Here's the drawing with two shaded views (mm, measured from the low corner). I have some questions. Round coordinates to 2 decimals unless told otherwise and drop trailing zeros. Loops run counter-clockwise (first coordinate to the right, second up) from the corner with the lowest first, then second, coordinate; pieces in that order, holes last.
(1) If I drill on line 1 along Y through (x, z) = (1.1, 88); line 2 along Y through (x, z) = (3.95, 91); line 3 along Z through (x, y) = (3.9, 36), over which ranges is the centre line in solid material (lowest first)?
(2) I want a section at A-A on z = 31. Write out the boundary of the cut face in (x, y).
(3) I want a section at D-D on y = 28.5. Write out the boundary of the cut face in (x, z).
(4) I want a section at B-B on z = 88. Write out the boundary of the cut face in (x, y), plus the area to 3 significant figures.
(5) Will these pins go through, and if not, where does the flat tip stop? pin 1 Ø1.5 at (x, z) = (2.5, 120.5) entering from -Y; pin 2 Ø5 at (y, z) = (64.5, 38) entering from -X; pin 3 Ø1.5 at (x, y) = (1.5, 77) entering from -Z; pin 4 Ø1.5 at (x, y) = (3.5, 78) entering from +Z.
(6) I want a section at C-C on x = 3.3. Give the number of separate pieces and of enclosed holes in the cut face, plus the area to 3 significant figures.
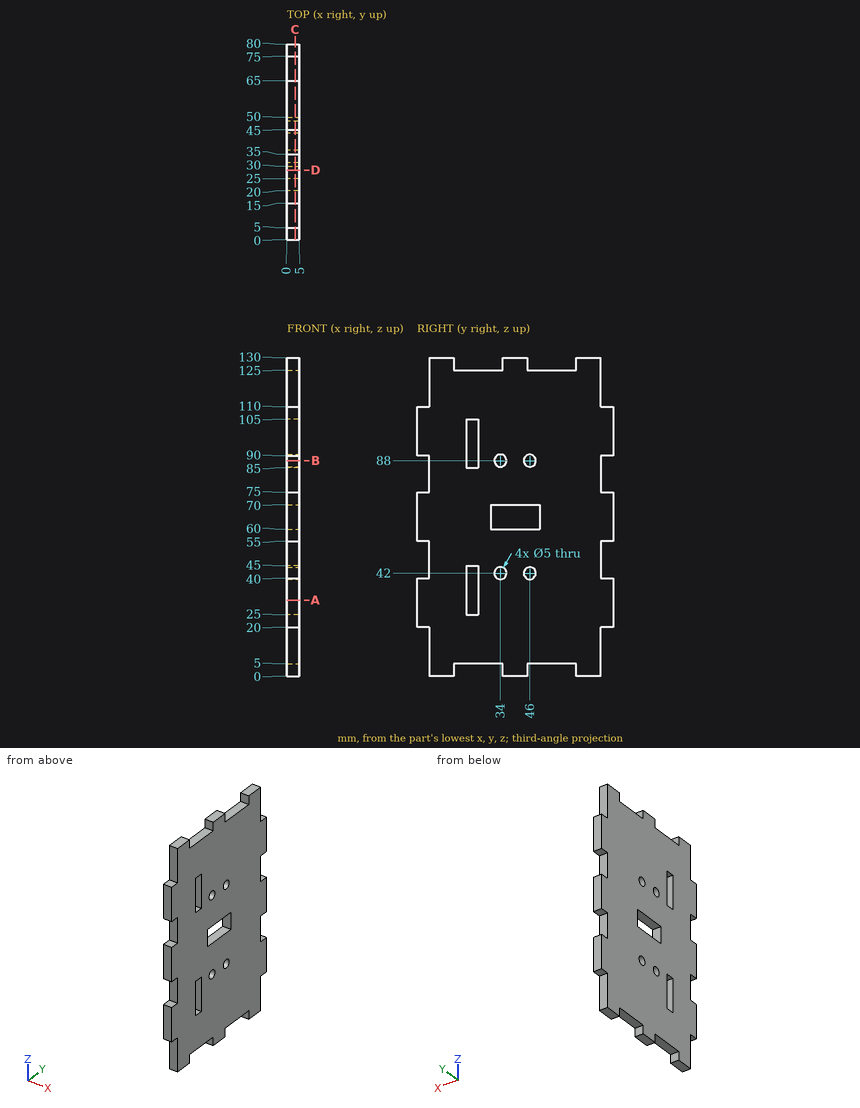
Filled sheet:
1. line 1: y = 5 to 20, 25 to 31.5, 36.5 to 43.5, 48.5 to 75
1. line 2: y = 0 to 20, 25 to 80
1. line 3: z = 0 to 40.5, 43.5 to 60, 70 to 86.5, 89.5 to 130
2. outline: (0, 0) - (5, 0) - (5, 20) - (0, 20) - close; (0, 25) - (5, 25) - (5, 80) - (0, 80) - close
3. outline: (0, 5) - (5, 5) - (5, 125) - (0, 125) - close
4. outline: (0, 5) - (5, 5) - (5, 20) - (0, 20) - close; (0, 25) - (5, 25) - (5, 31.5) - (0, 31.5) - close; (0, 36.5) - (5, 36.5) - (5, 43.5) - (0, 43.5) - close; (0, 48.5) - (5, 48.5) - (5, 75) - (0, 75) - close
4. area: 275 mm2
5. pin 1: stops at y = 5
5. pin 2: stops at x = 0
5. pin 3: stops at z = 20
5. pin 4: stops at z = 110
6. separate pieces: 1
6. enclosed holes: 7
6. area: 8,820 mm2
